Print and shaded views of the part. All mm, measured from the part's lowest x, y and z. A direction names the side the tool comes from. Give positions to 0.01 mm unless a question says otherwise; leave off trailing zeros. Order: outer loops, then holes, each group sorted by start corner. A loop starts at its lowest first (then second) coordinate and runs counter-clockwise, first axis right, second up. Notation, with made-up numbers: (21, 85) -> (58, 85) arc R19 ccw to (58, 98) -> close; hole circle Ø11 at (61.5, 1). An arc over 180 degrees is marked (long way). One line per question, with ' | ' between items. Start each with the question number.
(1) Cut at A-A (x = 2.5). Give the cut face in (y, z), then the cut area to 3 significant figures.
(2) Cut at B-B (y = 2.5). Give the cut face in (x, z).
(3) Pin check, flat tips, straight feed: pin 1 Ø1.5 at (y, z) = (3, 25.5) entering from -X; pin 2 Ø1.5 at (x, y) = (11, 2.5) entering from -Z; pin 3 Ø2.5 at (x, y) = (31.5, 3) entering from -Z. Stop position of each tip, or through.
(4) Drill centre lines: L1, parallel to Y at x = 2.5, z = 0.3; L2, parallel to X at y = 2.5, z = 0.3; L3, parallel to Z at x = 30, y = 0.6. Where is each one in solid material? Low to high. Write a range as from..to.
(5) Which spindle directions (+Z, -Z, +X, -X, +Y, -Y) get a long thin tool onto all of the face, cutting with end or side? Do the marked faces 1 and 2. Say none if no direction does.
(6) Cut at C-C (y = 4.2). Give the cut face in (x, z).
(7) Cut at D-D (x = 7). Give the cut face in (y, z).
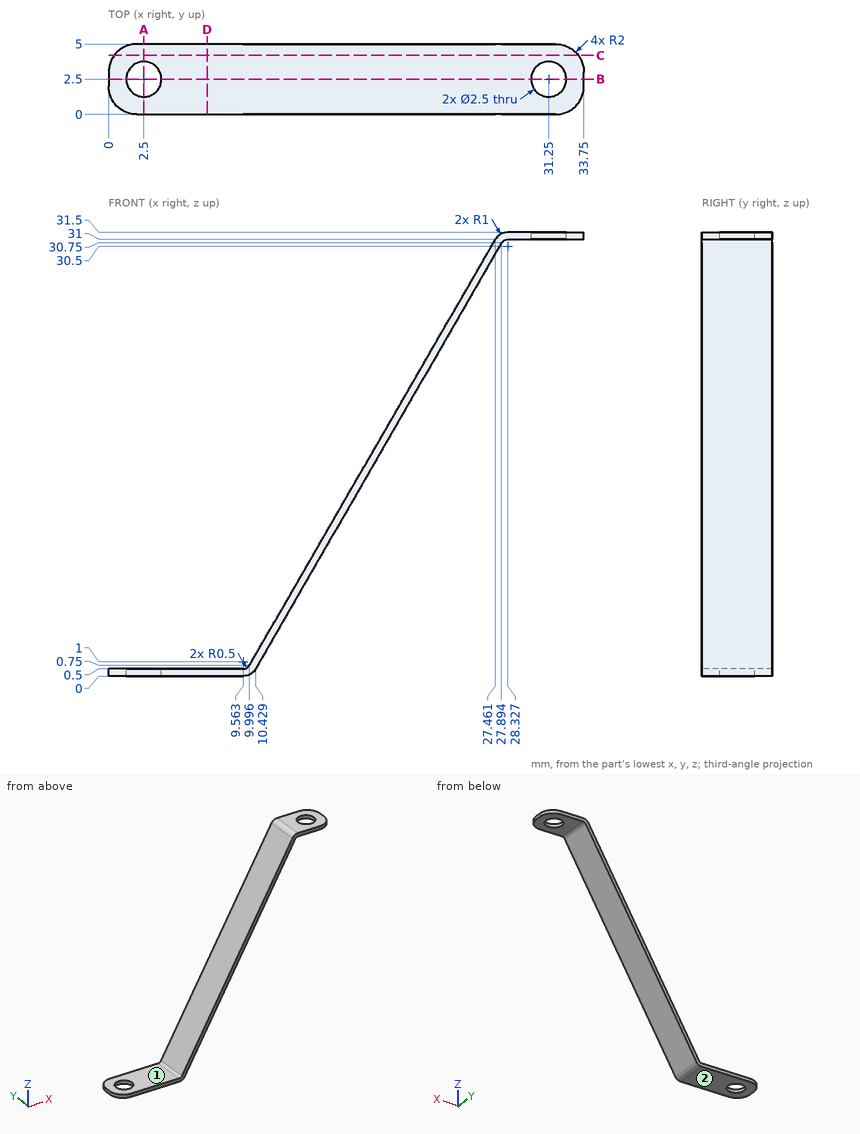
Result set:
1) outline: (0, 0) -> (1.25, 0) -> (1.25, 0.5) -> (0, 0.5) -> close; (3.75, 0) -> (5, 0) -> (5, 0.5) -> (3.75, 0.5) -> close | area: 1.25 mm2
2) outline: (0, 0) -> (1.25, 0) -> (1.25, 0.5) -> (0, 0.5) -> close; (3.75, 0) -> (9.56, 0) arc R1 ccw to (10.43, 0.5) -> (27.89, 30.75) arc R0.5 cw to (28.33, 31) -> (30, 31) -> (30, 31.5) -> (28.33, 31.5) arc R1 ccw to (27.46, 31) -> (10, 0.75) arc R0.5 cw to (9.56, 0.5) -> (3.75, 0.5) -> close; (32.5, 31) -> (33.75, 31) -> (33.75, 31.5) -> (32.5, 31.5) -> close
3) pin 1: stops at x = 23.85 | pin 2: stops at z = 0.27 | pin 3: stops at z = 31
4) L1: y = 0..1.25, 3.75..5 | L2: x = 0..1.25, 3.75..10.28 | L3: z = 31..31.5
5) face 1: +Z, -X, +Y, -Y | face 2: -Z, +X, -X, +Y, -Y
6) outline: (0.4, 0) -> (9.56, 0) arc R1 ccw to (10.43, 0.5) -> (27.89, 30.75) arc R0.5 cw to (28.33, 31) -> (33.35, 31) -> (33.35, 31.5) -> (28.33, 31.5) arc R1 ccw to (27.46, 31) -> (10, 0.75) arc R0.5 cw to (9.56, 0.5) -> (0.4, 0.5) -> close
7) outline: (0, 0) -> (5, 0) -> (5, 0.5) -> (0, 0.5) -> close
